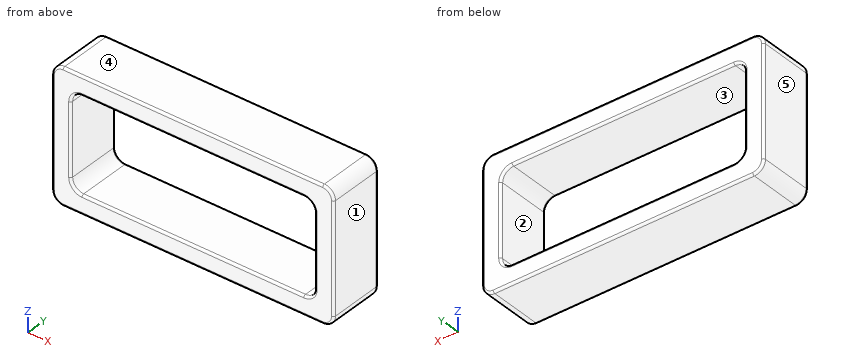
from build123d import *

# Parameters (mm, degrees)
F0_W     = 25.4
F0_H     = 11.9
F0_W_2   = 22
F0_H_2   = 8.5
F1_DEPTH = 5
F2_R     = 1
F3_R     = 0.2
F4_R     = 0.2


with BuildPart() as f1:
    # F0 (on Front) → F1 (new body)
    with BuildSketch(Plane.XZ):
        Rectangle(F0_W, F0_H)
        Rectangle(F0_W_2, F0_H_2, mode=Mode.SUBTRACT)
    extrude(amount=F1_DEPTH)

    # F2
    f2_edges = [f1.edges().sort_by_distance(p)[0] for p in [
        (-12.7, -2.5, 5.95),
        (12.7, -2.5, 5.95),
        (12.7, -2.5, -5.95),
        (-12.7, -2.5, -5.95),
        (-11, -2.5, 4.25),
        (-11, -2.5, -4.25),
        (11, -2.5, 4.25),
        (11, -2.5, -4.25),
    ]]
    fillet(f2_edges, radius=F2_R)

    # F3
    f3_edges = [f1.edges().sort_by_distance(p)[0] for p in [
        (0, 0, 5.95),
        (-12.407107, 0, 5.657107),
        (-12.7, 0, 0),
        (-12.407107, 0, -5.657107),
        (0, 0, -5.95),
        (12.407107, 0, -5.657107),
        (12.7, 0, 0),
        (12.407107, 0, 5.657107),
        (0, -5, -5.95),
        (12.7, -5, 0),
        (12.407107, -5, 5.657107),
        (0, -5, 5.95),
        (-12.407107, -5, 5.657107),
        (-12.7, -5, 0),
        (12.407107, -5, -5.657107),
        (-12.407107, -5, -5.657107),
    ]]
    fillet(f3_edges, radius=F3_R)

    # F4
    f4_edges = [f1.edges().sort_by_distance(p)[0] for p in [
        (0, 0, -4.25),
        (10.707107, 0, -3.957107),
        (11, 0, 0),
        (10.707107, 0, 3.957107),
        (0, 0, 4.25),
        (-11, 0, 0),
        (-10.707107, 0, -3.957107),
        (-10.707107, 0, 3.957107),
        (10.707107, -5, 3.957107),
        (10.707107, -5, -3.957107),
        (-10.707107, -5, -3.957107),
        (-11, -5, 0),
        (0, -5, 4.25),
        (11, -5, 0),
        (0, -5, -4.25),
    ]]
    fillet(f4_edges, radius=F4_R)


solid = f1.part
Geometry: final body of the model. Coordinates: model frame, mm. Face numbers are marked on the shaded views. A direction names the side the tool comes from. Give positions to 0.01 mm unless a question says otherwise; leave off trailing zeros. Loops run counter-clockwise (first coordinate to the right, second up) from the corner with the lowest first, then second, coordinate; pieces in that order, holes last. Notation, with made-up numbers: (44, -3.5) -> (84, -3.5) arc R24 cw to (84, 27.5) -> close; hole circle Ø8 at (51, 59). An arc over 180 degrees is marked (long way). Put each result on its own line as item: value.
1. Pull-direction query (X, two-part tool) for the marked faces 3, 4 and 5; classes: released by +X, released by -X, zero draft, split by the parting line, or undercut.
Taken from the geometry:
face 3: undercut
face 4: zero draft
face 5: released by -X
2. Cut plane C-C (z = -1.75). Return the cut outline in (x, y), plus the area to 3 significant figures.
Taken from the geometry:
outline: (-12.7, -4.8) arc R0.2 ccw to (-12.5, -5) -> (-11.2, -5) arc R0.2 ccw to (-11, -4.8) -> (-11, -0.2) arc R0.2 ccw to (-11.2, 0) -> (-12.5, 0) arc R0.2 ccw to (-12.7, -0.2) -> close; (11, -4.8) arc R0.2 ccw to (11.2, -5) -> (12.5, -5) arc R0.2 ccw to (12.7, -4.8) -> (12.7, -0.2) arc R0.2 ccw to (12.5, 0) -> (11.2, 0) arc R0.2 ccw to (11, -0.2) -> close
area: 16.9 mm2
3. Ray query, line 1 along Z through (x, y) = (-9.25, -2.35); line 2 along X through (y, z) = (-2, 3); line 3 along X through (y, z) = (-1.6, -3.75). Return the intervals inside material, ascending. Write a range as [from, to].
Taken from the geometry:
line 1: z = [-5.95, -4.25], [4.25, 5.95]
line 2: x = [-12.7, -11], [11, 12.7]
line 3: x = [-12.7, -10.87], [10.87, 12.7]
4. Pin query (flat end, axial travel): P1, Ø3, axis at x = 3.5, z = 2, coming from the +Y side. Return the tip coordinate at first contact, or that it passes through.
Taken from the geometry:
P1: passes through
5. Cut plane B-B (y = -3.6). Return the cut outline in (x, z), plus the area to 3 significant figures.
Taken from the geometry:
outline: (-12.7, -4.95) arc R1 ccw to (-11.7, -5.95) -> (11.7, -5.95) arc R1 ccw to (12.7, -4.95) -> (12.7, 4.95) arc R1 ccw to (11.7, 5.95) -> (-11.7, 5.95) arc R1 ccw to (-12.7, 4.95) -> close; hole (-11, -3.25) arc R1 ccw to (-10, -4.25) -> (10, -4.25) arc R1 ccw to (11, -3.25) -> (11, 3.25) arc R1 ccw to (10, 4.25) -> (-10, 4.25) arc R1 ccw to (-11, 3.25) -> close
area: 115 mm2
6. Cut plane A-A (x = -3.75). Return the cut outline in (y, z), plus the area to 3 significant figures.
Taken from the geometry:
outline: (-5, -5.75) arc R0.2 ccw to (-4.8, -5.95) -> (-0.2, -5.95) arc R0.2 ccw to (0, -5.75) -> (0, -4.45) arc R0.2 ccw to (-0.2, -4.25) -> (-4.8, -4.25) arc R0.2 ccw to (-5, -4.45) -> close; (-5, 4.45) arc R0.2 ccw to (-4.8, 4.25) -> (-0.2, 4.25) arc R0.2 ccw to (0, 4.45) -> (0, 5.75) arc R0.2 ccw to (-0.2, 5.95) -> (-4.8, 5.95) arc R0.2 ccw to (-5, 5.75) -> close
area: 16.9 mm2
7. Set-up query: the marked faces 1 and 2. Return all of +Z, -Z, +X, -X, +Y, -Y with unobstructed straight access to the full face (end or side cutting, diameter ignored); none if empty.
Taken from the geometry:
face 1: +Z, -Z, +X, +Y, -Y
face 2: +Y, -Y
